Part model, mm, in its own coordinate system. Face numbers are marked on the shaded views. Round coordinates to 2 decimals unless told otherwise and drop trailing zeros. Order: outer loops, then holes, each group sorted by start corner. A loop starts at its lowest first (then second) coordinate and runs counter-clockwise, first axis right, second up. Notation, with made-up numbers: (-7.5, 70.5) -> (18.5, 70.5) arc R28 ccw to (18.5, 106.5) -> close; hole circle Ø6 at (2.5, -28). An arc over 180 degrees is marked (long way). Answer as a JSON object with one key per item and string values. Group by question number.
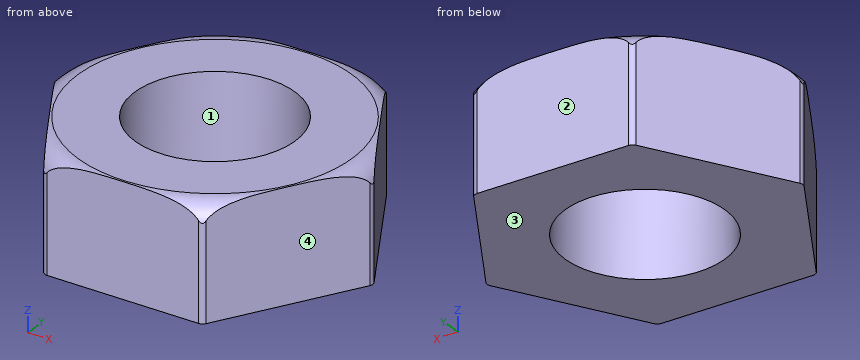
```python
from build123d import *

# Parameters (mm, degrees)
SKETCH1_R      = 3.175
EXTRUDE1_DEPTH = 2.2225
FILLET2_R      = 0.254


with BuildPart() as part:
    # Sketch1 → Extrude1 (new, symmetric)
    with BuildSketch(Plane.XY):
        Polygon((3.175, 5.499261314), (-3.175, 5.499261314), (-6.35, 0), (-3.175, -5.499261314), (3.175, -5.499261314), (6.35, 0), align=None)
        Circle(SKETCH1_R, mode=Mode.SUBTRACT)
    extrude(amount=EXTRUDE1_DEPTH, both=True)

    # Sketch7 → Cut-Revolve2 (revolve, cut)
    with BuildSketch(Plane(origin=(0, 0, 0), x_dir=(1, 0, 0), z_dir=(0, 1, 0)), mode=Mode.PRIVATE) as cut_revolve2_sk:
        with BuildLine():
            Line((5.310988996, -2.2225), (5.427200903, -2.2225))
            ThreePointArc((5.427200903, -2.2225), (6.079718402, -1.952218402), (6.35, -1.299700903))
            Line((6.35, -1.299700903), (6.71065175, -1.932108982))
            ThreePointArc((6.71065175, -1.932108982), (6.182957857, -2.514615502), (5.427200903, -2.7305))
            Line((5.427200903, -2.7305), (5.310988996, -2.7305))
            Line((5.310988996, -2.7305), (5.310988996, -2.2225))
        make_face()
    revolve(cut_revolve2_sk.sketch.rotate(Axis((0, 0, -4.413769038), (0, 0, 1)), 180), axis=Axis((0, 0, -4.413769038), (0, 0, 1)), mode=Mode.SUBTRACT)

    # Fillet2
    # the kernel refuses this fillet: 0.254 mm, written as the material it takes off along each edge
    with BuildSketch(Plane(origin=(-3.175, 5.499261314, -2.589117421), x_dir=(1, 0, 0), z_dir=(0, 0, 1)), Plane(origin=(3.175, 5.499261314, 1.666318324), x_dir=(-1, 0, 0), z_dir=(0, 0, -1)), Plane(origin=(6.35, 0, 1.666318324), x_dir=(-0.5000000000000007, 0.8660254037844384, 0), z_dir=(0, 0, -1)), Plane(origin=(3.175, -5.499261314, 1.666318324), x_dir=(0.49999999999999906, 0.8660254037844392, 0), z_dir=(0, 0, -1)), Plane(origin=(-3.175, -5.499261314, -2.589117421), x_dir=(-0.4999999999999997, 0.8660254037844387, 0), z_dir=(0, 0, 1)), Plane(origin=(-6.35, 0, -2.589117421), x_dir=(0.4999999999999968, 0.8660254037844406, 0), z_dir=(0, 0, 1))) as fillet2_piece_1:
        with BuildLine():
            CenterArc((FILLET2_R * 0.57735026919, -FILLET2_R), FILLET2_R, 90, 60)
            Line((-FILLET2_R * 0.288675134595, -FILLET2_R * 0.5), (0, 0))
            Line((0, 0), (FILLET2_R * 0.57735026919, 0))
        make_face()
    extrude(amount=4.255435745, mode=Mode.SUBTRACT)


solid = part.part
```
Q1. Wall check: line 1 (Y direction, x = 0, z = 1) (3 decimals); line 2 (Y direction, x = 0.75, z = 1.05); line 3 (X direction, y = -2.5, z = -1.45). Give the ranges that are in metal, low to high. Write a range as [from, to].
Q2. Band-saw the part on C-C (z = 1.8). List the corners of the cut face in (x, y) (3 decimals).
Q3. Band-saw the part on B-B (z = 1.15). List the corners of the cut face in (x, y) (3 decimals).
Q4. Drop a flat-ended pin along its axis: pin 1 Ø2 at (y, z) = (-4, -1) entering from -X. Give the stop position or say it passes through.
Q5. Two-plate mould, pull along Y, no slides. Class the marked faces 1, 2, 3 and 4: +Y half, -Y half, draft (parallel to the pull), parting line (faces both ways), or undercut.
Completed:
{
 "1": {"line 1": "[-5.499, -3.175], [3.175, 5.499]", "line 2": "[-5.5, -3.09], [3.09, 5.5]", "line 3": "[-4.91, -1.96], [1.96, 4.91]"},
 "2": {"outline": "(-6.197, -0.265) -> (-3.328, -5.234) arc R6.203 ccw to (-2.869, -5.499) -> (2.869, -5.499) arc R6.203 ccw to (3.328, -5.234) -> (6.197, -0.265) arc R6.203 ccw to (6.197, 0.265) -> (3.328, 5.234) arc R6.203 ccw to (2.869, 5.499) -> (-2.869, 5.499) arc R6.203 ccw to (-3.328, 5.234) -> (-6.197, 0.265) arc R6.203 ccw to start; hole circle Ø6.35 at (0, 0)"},
 "3": {"outline": "(-6.277, -0.127) -> (-3.248, -5.372) arc R0.254 ccw to (-3.028, -5.499) -> (3.028, -5.499) arc R0.254 ccw to (3.248, -5.372) -> (6.277, -0.127) arc R0.254 ccw to (6.277, 0.127) -> (3.248, 5.372) arc R0.254 ccw to (3.028, 5.499) -> (-3.028, 5.499) arc R0.254 ccw to (-3.248, 5.372) -> (-6.277, 0.127) arc R0.254 ccw to start; hole circle Ø6.35 at (0, 0)"},
 "4": {"pin 1": "x = -4.62"},
 "5": {"face 1": "undercut", "face 2": "+Y half", "face 3": "draft", "face 4": "-Y half"}
}
